from build123d import *

# Parameters (mm, degrees)
EXTRUDE_1_DEPTH = 4
CHAMFER_1_SIZE  = 1
SKETCH_2_R      = 2.1
EXTRUDE_2_DEPTH = 3


with BuildPart() as part:
    # 草图1 → 拉伸1 (new body)
    with BuildSketch(Plane(origin=(0, 0, 0), x_dir=(1, 0, 0), z_dir=(0, 1, 0))):
        Polygon((4.174188702, -3.988669204), (5.541383209, 1.620618854), (1.367194507, 5.609288058), (-4.174188702, 3.988669204), (-5.541383209, -1.620618854), (-1.367194507, -5.609288058), align=None)
    extrude(amount=EXTRUDE_1_DEPTH)

    # 倒角1
    chamfer_1_edges = [part.edges().sort_by_distance(p)[0] for p in [
        (3.454288858, 4, -3.614953456),
        (-1.403497097, 4, -4.798978631),
        (-4.857785955, 4, -1.184025175),
        (-3.454288858, 4, 3.614953456),
        (1.403497097, 4, 4.798978631),
        (4.857785955, 4, 1.184025175),
    ]]
    chamfer(chamfer_1_edges, length=CHAMFER_1_SIZE)

    # 草图2 → 拉伸2 (add)
    with BuildSketch(Plane.XZ):
        with Locations(Location((0, 0, 0), (0, 0, 90))):
            Circle(SKETCH_2_R)
    extrude(amount=EXTRUDE_2_DEPTH)


solid = part.part
Source: CAD feature listing. Evaluate the final solid. Frame: model axes, mm. A direction names the side the tool comes from. Give positions to 0.01 mm unless a question says otherwise; leave off trailing zeros. Write each loop counter-clockwise with the first axis right and the second up, starting at its lowest first coordinate (ties: lowest second). Pieces come first, ordered by that corner, then holes. Notation, with made-up numbers: M 28,68.25 L 60,68.25 A4 cw 60,72.25 Z; hole C 58,61.25 d10. An arc over 180 degrees is marked long. Answer as a JSON object with one key per item and string values.
Q1. Cut plane D-D, the plane x = -2.75. Return the cut outline in (y, z), then the cut area to 3 significant figures.
Geometry check:
{"outline": "M 0,-4.41 L 3,-4.41 L 4,-3.36 L 4,2.9 L 3,4.29 L 0,4.29 Z", "area": "33.6 mm^2"}
Q2. Cut plane A-A, the plane y = 0.25. Return the cut outline in (x, z).
Geometry check:
{"outline": "M -5.54,1.62 L -4.17,-3.99 L 1.37,-5.61 L 5.54,-1.62 L 4.17,3.99 L -1.37,5.61 Z"}
Q3. Cut plane C-C, the plane x = 0. Return the cut outline in (y, z), then the cut area to 3 significant figures.
Geometry check:
{"outline": "M -3,-2.1 L 0,-2.1 L 0,-5.21 L 3,-5.21 L 4,-4.17 L 4,4.17 L 3,5.21 L 0,5.21 L 0,2.1 L -3,2.1 Z", "area": "53.2 mm^2"}
Q4. Contact query for flat-ended pins moving along their axis: P1, Ø1.5, axis at y = 2.5, z = 2.5, coming from the +X side; P2, Ø1, axis at x = -2.5, z = 4, coming from the +Y side; P3, Ø1.5, axis at x = 4.5, z = -3, coming from the -Y side. Output: stop coordinate, or through.
Geometry check:
{"P1": "stops at x = 4.72", "P2": "stops at y = 3.88", "P3": "stops at y = 0"}
Q5. Cut plane B-B, the plane z = 0. Return the cut outline in (x, y).
Geometry check:
{"outline": "M -5.15,0 L -2.1,0 L -2.1,-3 L 2.1,-3 L 2.1,0 L 5.15,0 L 5.15,3 L 4.12,4 L -4.12,4 L -5.15,3 Z"}
Q6. Access query for faces 1 (the face through (-0.631, -1.479, 2.003)), 2 (the face through (-4.356, 3.507, -1.103)). Directions: +Z, -Z, +X, -X, +Y, -Y. A direction counts if a zero-diameter tool reaches every point of the face in a straight line with its end or side. Return the directions, or none.
Geometry check:
{"face 1": "-Y", "face 2": "-Z, -X, +Y"}
Q7. Ray query, line 1 along Y through (x, z) = (3.5, -1); line 2 along X through (y, z) = (-1.5, 0); line 3 along Z through (x, y) = (-1.5, 1). Return the intervals inside material, ascending.
Geometry check:
{"line 1": "y = 0 to 4", "line 2": "x = -2.1 to 2.1", "line 3": "z = -4.77 to 5.48"}
